```python
from build123d import *
from build123d.topology import SkipClean

# Parameters (mm, degrees)
BOSS_EXTRUDE1_DEPTH = 6.35
CHAMFER1_SIZE       = 3.175
BOSS_EXTRUDE2_DEPTH = 12.7
CHAMFER2_SIZE       = 12.7
CHAMFER3_SIZE       = 6.35
SKETCH3_W           = 90.7
SKETCH3_H           = 45.44
CUT_EXTRUDE1_DEPTH  = 9.47
BOSS_EXTRUDE3_DEPTH = 24.5
CHAMFER4_SIZE       = 6.35
SKETCH5_R           = 1.35
CUT_EXTRUDE2_DEPTH  = 24.5
FILLET1_R           = 2.5
SKETCH6_W           = 58.4
SKETCH6_H           = 26.5
BOSS_EXTRUDE4_DEPTH = 3.23
SKETCH7_R           = 2.5
CUT_EXTRUDE4_DEPTH  = 12.7
SKETCH8_R           = 1.35
CUT_EXTRUDE5_DEPTH  = 89.292426062


with BuildPart() as part:
    # Sketch1 → Boss-Extrude1 (new body)
    with BuildSketch(Plane(origin=(0, 0, 0), x_dir=(0, 0, -1), z_dir=(1, 0, 0))):
        Polygon((-64.4, -46.35), (-64.4, 59.05), (64.4, 59.05), (64.4, -46.35), (51.7, -46.35), (51.7, 46.35), (-51.7, 46.35), (-51.7, -46.35), align=None)
    extrude(amount=BOSS_EXTRUDE1_DEPTH)

    # Chamfer1
    chamfer1_edges = [part.edges().sort_by_distance(p)[0] for p in [
        (6.35, 6.35, -64.4),
        (6.35, 59.05, 0),
        (6.35, 6.35, 64.4),
    ]]
    chamfer(chamfer1_edges, length=CHAMFER1_SIZE)

    # Sketch2 → Boss-Extrude2 (add)
    with BuildSketch(Plane(origin=(6.35, 0, 0), x_dir=(0, 0, -1), z_dir=(1, 0, 0))):
        Polygon((-51.7, -5.44), (-31.2, -5.44), (-31.2, 35.96), (27.2, 35.96), (27.2, -5.44), (51.7, -5.44), (51.7, 46.35), (-51.7, 46.35), align=None)
        Polygon((-61.225, -5.44), (-51.7, -5.44), (-51.7, 46.35), (51.7, 46.35), (51.7, -5.44), (61.225, -5.44), (61.225, 55.875), (-61.225, 55.875), align=None)
    extrude(amount=BOSS_EXTRUDE2_DEPTH)

    # Chamfer2
    chamfer2_edges = [part.edges().sort_by_distance(p)[0] for p in [
        (19.05, 25.2175, -61.225),
        (19.05, 55.875, 0),
        (19.05, 25.2175, 61.225),
    ]]
    chamfer(chamfer2_edges, length=CHAMFER2_SIZE - 0.0001)  # a hair under: the kernel refuses the full size

    # Chamfer3
    chamfer3_edges = [part.edges().sort_by_distance(p)[0] for p in [
        (6.35, 20.455, -51.7),
        (6.35, 46.35, 0),
        (6.35, 20.455, 51.7),
    ]]
    chamfer(chamfer3_edges, length=CHAMFER3_SIZE - 0.0001)  # a hair under: the kernel refuses the full size

    # Sketch3 → Cut-Extrude1 (cut)
    with BuildSketch(Plane.ZY.offset(-6.35)):
        with Locations((0, 17.28)):
            Rectangle(SKETCH3_W, SKETCH3_H)
    extrude(amount=-CUT_EXTRUDE1_DEPTH, mode=Mode.SUBTRACT)

    # Sketch4 → Boss-Extrude3 (add)
    with SkipClean():  # the faces are left unmerged after this step: merging them gives an invalid solid
        with BuildSketch(Plane.XZ.offset(5.44)):
            Polygon((15.82, -27.2), (15.82, -45.35), (6.35, -45.35), (0, -51.7), (6.35, -51.7), (6.35, -61.225), (19.05, -48.525), (19.05, -27.2), align=None)
            Polygon((0, 51.7), (6.35, 45.35), (15.82, 45.35), (15.82, 31.2), (19.05, 31.2), (19.05, 48.525), (6.35, 61.225), (6.35, 51.7), align=None)
        extrude(amount=BOSS_EXTRUDE3_DEPTH)

    # Chamfer4
    chamfer4_edges = [part.edges().sort_by_distance(p)[0] for p in [
        (6.35, -46.35, -56.4625),
        (6.35, -46.35, 56.4625),
    ]]
    chamfer(chamfer4_edges, length=CHAMFER4_SIZE - 0.0001)  # a hair under: the kernel refuses the full size

    # Sketch5 → Cut-Extrude2 (cut)
    with SkipClean():  # the faces are left unmerged after this step: merging them gives an invalid solid
        with BuildSketch(Plane(origin=(6.35, 0, 0), x_dir=(0, 0, -1), z_dir=(1, 0, 0))):
            with Locations((-56.4625, -34.97)):
                Circle(SKETCH5_R)
            with Locations((56.4625, -34.97)):
                Circle(SKETCH5_R)
        extrude(amount=-CUT_EXTRUDE2_DEPTH, mode=Mode.SUBTRACT)

    # Fillet1
    fillet1_edges = [part.edges().sort_by_distance(p)[0] for p in [
        (3.175, 7.93745, 64.4),
        (3.175, 7.93745, -64.4),
        (3.175, 59.05, 0),
    ]]
    fillet(fillet1_edges, radius=FILLET1_R)

    # Sketch6 → Boss-Extrude4 (add)
    with SkipClean():  # the faces are left unmerged after this step: merging them gives an invalid solid
        with BuildSketch(Plane(origin=(19.05, 0, 0), x_dir=(0, 0, -1), z_dir=(1, 0, 0))):
            with Locations((-2, -16.69)):
                Rectangle(SKETCH6_W, SKETCH6_H)
        extrude(amount=-BOSS_EXTRUDE4_DEPTH)

    # Sketch7 → Cut-Extrude4 (cut)
    with SkipClean():  # the faces are left unmerged after this step: merging them gives an invalid solid
        with BuildSketch(Plane(origin=(19.05, 0, 0), x_dir=(0, 0, -1), z_dir=(1, 0, 0))):
            with Locations(Location((-56.4625, 51.1125, 0), (0, 0, 315))):
                Circle(SKETCH7_R)
            with Locations(Location((56.4625, 51.1125, 0), (0, 0, 45))):
                Circle(SKETCH7_R)
        extrude(amount=-CUT_EXTRUDE4_DEPTH, mode=Mode.SUBTRACT)

    # Sketch8 → Cut-Extrude5 (cut, through all)
    with SkipClean():  # the faces are left unmerged after this step: merging them gives an invalid solid
        with BuildSketch(Plane(origin=(6.35, 0, 0), x_dir=(0, 0, -1), z_dir=(1, 0, 0))):
            with Locations((-56.4625, 51.1125)):
                Circle(SKETCH8_R)
            with Locations((56.4625, 51.1125)):
                Circle(SKETCH8_R)
        extrude(amount=-CUT_EXTRUDE5_DEPTH, mode=Mode.SUBTRACT)


solid = part.part
```
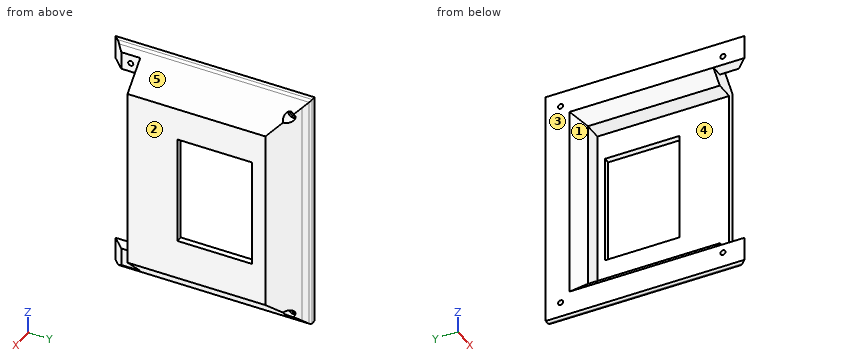
CAD build for the part. Positions are in the model's coordinates, mm. Face numbers are marked on the shaded views. A direction names the side the tool comes from. Round coordinates to 2 decimals unless told otherwise and drop trailing zeros.
Item 1: Saw through at B-B on y = -34.97. State how many separate pieces and enclosed holes the cut face has, then the cut area to 3 significant figures.
Item 2: Tool access for the marked faces 1 and 2: list every direction of +Z, -Z, +X, -X, +Y, -Y with a clear straight run to the whole face (end or side of a thin tool).
Item 3: Pin check, flat tips, straight feed: pin 1 (1.5 mm diameter, centred on y = 50, z = 57, fed in from +X); pin 2 (1 mm diameter, centred on x = 18, z = 8, fed in from -Y); pin 3 (4 mm diameter, centred on x = 15.5, y = 13.5, fed in from +Z) (3 decimals). Stop position of each tip, or through.
Item 4: Probe line 1 along Z through (x, y) = (10.25, -28) (3 decimals); line 2 along Z through (x, y) = (9, 15) (3 decimals); line 3 along X through (y, z) = (38, -18). List the from-to ranges inside material, lowest first.
Item 5: Mould opens along Z. For the marked faces 3, 4 and 5 say: pulls with the +Z half, pulls with the -Z half, needs draft (parallel to the pull), parting line crosses it, or undercut.
Reported:
1. separate pieces: 4
1. enclosed holes: 0
1. area: 117 mm2
2. face 1: -X, -Y
2. face 2: +Z, -Z, +X, +Y, -Y
3. pin 1: stops at x = 6.35
3. pin 2: stops at y = -29.94
3. pin 3: stops at z = 54.075
4. line 1: z = -57.325 to -45.35, 45.35 to 57.325
4. line 2: z = -58.575 to -45.35, 45.35 to 58.575
4. line 3: x = 15.82 to 19.05
5. face 3: needs draft
5. face 4: undercut
5. face 5: pulls with the +Z half
